Build history of the part. All positions in model axes, mm. A direction names the side the tool comes from. Give positions to 0.01 mm unless a question says otherwise; leave off trailing zeros. Write each loop counter-clockwise with the first axis right and the second up, starting at its lowest first coordinate (ties: lowest second). Pieces come first, ordered by that corner, then holes. Notation, with made-up numbers: (79, 1.25) -> (114, 1.25) arc R21 ccw to (114, 29.25) -> close; hole circle Ø3 at (53.25, 8.25). An arc over 180 degrees is marked (long way). Put each result on its own line as item: value. Start each with the question number.
Item 1: Two-plate mould, pull along Y, no slides. Class faces 4 (the flat face through (-1, 39, -57)), 5 (the flat face through (-105.938, 65.362, -81.367)), 6 (the flat face through (-56, 40, -85)): pulls with the +Y half, pulls with the -Y half, needs draft (parallel to the pull), parting line crosses it, or undercut.
Item 2: Flat gauge pins, fed straight in: pin 1 Ø3 at (x, y) = (-90.5, 63.5) entering from +Z; pin 2 Ø1.1 at (x, y) = (-0.5, 57.5) entering from -Z; pin 3 Ø0.8 at (x, y) = (-93, -0.5) entering from +Z. Where does each tip first touch, or does it go through?
Item 3: Drill centre lines: line 1 along X through (y, z) = (25.5, -52.5); line 2 along Y through (x, z) = (-59, -66); line 3 along X through (y, z) = (79.7, -60). Where is each one in solid material? Low to high.
Item 4: Slice it at A-A, the plane z = -60. List the corners of the cut face in (x, y), plus the area to 3 significant figures.
Item 5: Slice it at C-C, the plane y = 34. List the corners of the cut face in (x, z), plus the area to 3 significant figures.
Item 6: Slice it at D-D, the plane x = -38.5. List the corners of the cut face in (y, z), plus the area to 3 significant figures.
Item 7: Tool access for faces 1 (the flat face through (-106.823, 40.053, -14.629)), 2 (the cylindrical face through (-50.043, 79.507, -60.651)), 3 (the flat face through (-5.938, 69.54, -81.574)): list every direction of +Z, -Z, +X, -X, +Y, -Y with a clear straight run to the whole face (end or side of a thin tool).
Item 8: Slice it at B-B, the plane x = -52. List the corners of the cut face in (y, z).
```python
from build123d import *
from OCP.BRepFilletAPI import BRepFilletAPI_MakeChamfer

# Parameters (mm, degrees)
SKETCH_1_W                 = 110
SKETCH_1_H                 = 85
EXTRUDE_1_DEPTH            = 80
CUT_EXTRUDE_1_REACH        = 162.39
CHAMFER_1_SIZE             = 5
CHAMFER_1_SIZE2            = 10
SPLIT_START                = 61.095980997
SPLIT_BODIES_3_OUTLINE_W   = 98
SPLIT_BODIES_3_OUTLINE_H   = 75
SPLIT_BODIES_3_DEPTH       = 8.1461308
SPLIT_START_2              = -128.980404327
SPLIT_BODIES_3_2_OUTLINE_W = 98
SPLIT_BODIES_3_2_OUTLINE_H = 75
SPLIT_BODIES_3_2_DEPTH     = 8.146130799
SPLIT_START_3              = -145.272665927
SPLIT_BODIES_3_3_OUTLINE_W = 98
SPLIT_BODIES_3_3_OUTLINE_H = 76
SPLIT_BODIES_3_3_DEPTH     = 8.1461308
SPLIT_START_4              = 77.388242596
SPLIT_BODIES_3_4_OUTLINE_W = 99
SPLIT_BODIES_3_4_OUTLINE_H = 76
SPLIT_BODIES_3_4_DEPTH     = 8.1461308
SHELL_2_T                  = -1
SKETCH_6_R                 = 5
CUT_EXTRUDE_2_DEPTH        = 10
SKETCH_7_W                 = 21
SKETCH_7_H                 = 41
CUT_EXTRUDE_3_DEPTH        = 161.390149323
EXTRUDE_2_DEPTH            = 1
SKETCH_9_W                 = 21
SKETCH_9_H                 = 41
CUT_EXTRUDE_5_DEPTH        = 1


# Read off the part's stored shape, not the designer's step: 分割3
with BuildPart() as part:
    # 草图1 → 凸台-拉伸1 (new body)
    with BuildSketch(Plane(origin=(0, 0, 0), x_dir=(1, 0, 0), z_dir=(0, 1, 0))):
        with Locations((-55, 42.5)):
            Rectangle(SKETCH_1_W, SKETCH_1_H)
    extrude(amount=EXTRUDE_1_DEPTH)

    # 草图2 → 切除-拉伸1 (cut, up to next)
    with BuildSketch(Plane(origin=(0, 80, 0), x_dir=(1, 0, 0), z_dir=(0, 1, 0)), mode=Mode.PRIVATE) as cut_extrude_1_sk1:
        Polygon((-85, 0), (-110, 10), (-110, 0), align=None)
    cut_extrude_1_tool1 = extrude(cut_extrude_1_sk1.sketch, amount=-CUT_EXTRUDE_1_REACH, mode=Mode.PRIVATE) & part.part
    # 草图2 → 切除-拉伸1 (cut, up to next)
    with BuildSketch(Plane(origin=(0, 80, 0), x_dir=(1, 0, 0), z_dir=(0, 1, 0)), mode=Mode.PRIVATE) as cut_extrude_1_sk2:
        Polygon((0, 10), (-25, 0), (0, 0), align=None)
    cut_extrude_1_tool2 = extrude(cut_extrude_1_sk2.sketch, amount=-CUT_EXTRUDE_1_REACH, mode=Mode.PRIVATE) & part.part
    add(cut_extrude_1_tool1.solids().sort_by_distance((-101.666667, 80, -3.333333))[0], mode=Mode.SUBTRACT)
    add(cut_extrude_1_tool2.solids().sort_by_distance((-8.333333, 80, -3.333333))[0], mode=Mode.SUBTRACT)

    # Split Bodies 2
    split(bisect_by=Plane(origin=(0, 5.030044473, 13.819933608), x_dir=(0, 0.9396926207859094, -0.3420201433256661), z_dir=(0, 0.3420201433256661, 0.9396926207859094)), keep=Keep.BOTTOM)

    # 倒角1: one chamfer whose edges measure the first distance from different faces: ONE call of the kernel's chamfer builder (chamfer() names one face for all edges)
    chamfer_1_edges_1 = [part.edges().sort_by_distance(p)[0] for p in [
        (-110, 35.237387097, -10),
    ]]
    chamfer_1_side_1 = [part.faces().sort_by_distance(p)[0] for p in [
        (-98.508842949, 28.923048193, -5.40353718),
    ]]
    chamfer_1_edges_2 = [part.edges().sort_by_distance(p)[0] for p in [
        (0, 35.237387097, -10),
    ]]
    chamfer_1_side_2 = [part.faces().sort_by_distance(p)[0] for p in [
        (0, 39.898381252, -47.600292644),
    ]]
    chamfer_1 = BRepFilletAPI_MakeChamfer(part.part.solid().wrapped)
    for e in chamfer_1_edges_1:
        chamfer_1.Add(CHAMFER_1_SIZE, CHAMFER_1_SIZE2, e.wrapped, chamfer_1_side_1[0].wrapped)  # the first distance lies on this face
    for e in chamfer_1_edges_2:
        chamfer_1.Add(CHAMFER_1_SIZE, CHAMFER_1_SIZE2, e.wrapped, chamfer_1_side_2[0].wrapped)  # the first distance lies on this face
    add(Compound.cast(chamfer_1.Shape()), mode=Mode.REPLACE)

    # Split Bodies 3 outline → Split Bodies 3 (cut)
    with BuildSketch(Plane(origin=(0, 0, 0), x_dir=(0.839683943173837, 0.13171512834099375, 0.5268605133639755), z_dir=(0.5430753866417041, -0.20365326999063904, -0.8146130799625572)).offset(SPLIT_START)):
        with Locations((-79, -54.5)):
            Rectangle(SPLIT_BODIES_3_OUTLINE_W, SPLIT_BODIES_3_OUTLINE_H)
    extrude(amount=SPLIT_BODIES_3_DEPTH, mode=Mode.SUBTRACT)

    # Split Bodies 3 2 outline → Split Bodies 3 2 (cut)
    with BuildSketch(Plane(origin=(0, 0, 0), x_dir=(0.8396839431738365, -0.13171512834099394, -0.5268605133639763), z_dir=(0.5430753866417047, 0.20365326999063899, 0.8146130799625568)).offset(SPLIT_START_2)):
        with Locations((-13, 54.5)):
            Rectangle(SPLIT_BODIES_3_2_OUTLINE_W, SPLIT_BODIES_3_2_OUTLINE_H)
    extrude(amount=SPLIT_BODIES_3_2_DEPTH, mode=Mode.SUBTRACT)

    # Split Bodies 3 3 outline → Split Bodies 3 3 (cut)
    with BuildSketch(Plane(origin=(0, 0, 0), x_dir=(0.8396839431738365, 0.13171512834099394, -0.5268605133639763), z_dir=(0.5430753866417047, -0.20365326999063899, 0.8146130799625568)).offset(SPLIT_START_3)):
        with Locations((-2, 23)):
            Rectangle(SPLIT_BODIES_3_3_OUTLINE_W, SPLIT_BODIES_3_3_OUTLINE_H)
    extrude(amount=SPLIT_BODIES_3_3_DEPTH, mode=Mode.SUBTRACT)

    # Split Bodies 3 4 outline → Split Bodies 3 4 (cut)
    with BuildSketch(Plane(origin=(0, 0, 0), x_dir=(0.839683943173837, -0.13171512834099375, 0.5268605133639755), z_dir=(0.5430753866417041, 0.20365326999063904, -0.8146130799625572)).offset(SPLIT_START_4)):
        with Locations((-89.5, -23)):
            Rectangle(SPLIT_BODIES_3_4_OUTLINE_W, SPLIT_BODIES_3_4_OUTLINE_H)
    extrude(amount=SPLIT_BODIES_3_4_DEPTH, mode=Mode.SUBTRACT)

    # 抽壳2
    shell_2_openings = [part.faces().sort_by_distance(p)[0] for p in [
        (-54.995965718, 0, -43.10116127),
    ]]
    offset(amount=SHELL_2_T, openings=shell_2_openings, kind=Kind.INTERSECTION)

    # 草图6 → 切除-拉伸2 (cut)
    with BuildSketch(Plane(origin=(0, 80, 0), x_dir=(1, 0, 0), z_dir=(0, 1, 0))):
        with Locations(Location((-55, 60, 0), (0, 0, 270))):
            Circle(SKETCH_6_R)
    extrude(amount=-CUT_EXTRUDE_2_DEPTH, mode=Mode.SUBTRACT)

    # 草图7 → 切除-拉伸3 (cut, through all)
    with BuildSketch(Plane(origin=(0, 0, 0), x_dir=(0, 0, -1), z_dir=(1, 0, 0))):
        with Locations((41.5, 48.5)):
            Rectangle(SKETCH_7_W, SKETCH_7_H)
    extrude(amount=-CUT_EXTRUDE_3_DEPTH, mode=Mode.SUBTRACT)

    # 草图8 → 凸台-拉伸2 (add)
    with BuildSketch(Plane.XZ):
        Polygon((-110, -75), (-95, -85), (-15, -85), (0, -75), (0, -15), (-9.284766909, -6.286093236), (-25, 0), (-85, 0), (-105.357616546, -8.143046618), (-110, -20), align=None)
    extrude(amount=EXTRUDE_2_DEPTH)

    # 草图9 → 切除-拉伸5 (cut)
    with BuildSketch(Plane.XZ.offset(1)):
        with Locations((-20.5, -49.5)):
            Rectangle(SKETCH_9_W, SKETCH_9_H)
        with Locations((-89.5, -49.5)):
            Rectangle(SKETCH_9_W, SKETCH_9_H)
    extrude(amount=-CUT_EXTRUDE_5_DEPTH, mode=Mode.SUBTRACT)


solid = part.part
```
Values follow:
1. face 4: undercut
1. face 5: pulls with the +Y half
1. face 6: needs draft
2. pin 1: z = -6.92
2. pin 2: z = -81.35
2. pin 3: z = -3.04
3. line 1: -110 to -109, -1 to 0
3. line 2: -1 to 0, 79 to 80
3. line 3: -110 to -60, -50 to 0
4. outline: (-110, -1) -> (-100, -1) -> (-100, 0) -> (-109, 0) -> (-109, 79) -> (-60, 79) -> (-60, 80) -> (-110, 80) -> close; (-79, -1) -> (-31, -1) -> (-31, 0) -> (-79, 0) -> close; (-50, 79) -> (-1, 79) -> (-1, 0) -> (-10, 0) -> (-10, -1) -> (0, -1) -> (0, 80) -> (-50, 80) -> close
4. area: 326 mm2
5. outline: (-110, -83.5) -> (-107.75, -85) -> (-2.25, -85) -> (0, -83.5) -> (0, -52) -> (-1, -52) -> (-1, -82.94) -> (-2.59, -84) -> (-107.41, -84) -> (-109, -82.94) -> (-109, -52) -> (-110, -52) -> close; (-110, -31) -> (-109, -31) -> (-109, -20.19) -> (-104.58, -8.91) -> (-84.81, -1) -> (-25.19, -1) -> (-9.83, -7.14) -> (-1, -15.43) -> (-1, -31) -> (0, -31) -> (0, -15) -> (-9.28, -6.29) -> (-25, 0) -> (-85, 0) -> (-105.36, -8.14) -> (-110, -20) -> close
5. area: 322 mm2
6. outline: (-1, -85) -> (80, -85) -> (80, -13.47) -> (43, 0) -> (-1, 0) -> close; hole (0, -84) -> (79, -84) -> (79, -14.17) -> (42.82, -1) -> (0, -1) -> close
6. area: 317 mm2
7. face 1: none
7. face 2: +Y
7. face 3: -Z, +X, +Y
8. outline: (-1, -85) -> (80, -85) -> (80, -64) -> (79, -64) -> (79, -84) -> (0, -84) -> (0, -1) -> (42.82, -1) -> (79, -14.17) -> (79, -56) -> (80, -56) -> (80, -13.47) -> (43, 0) -> (-1, 0) -> close
